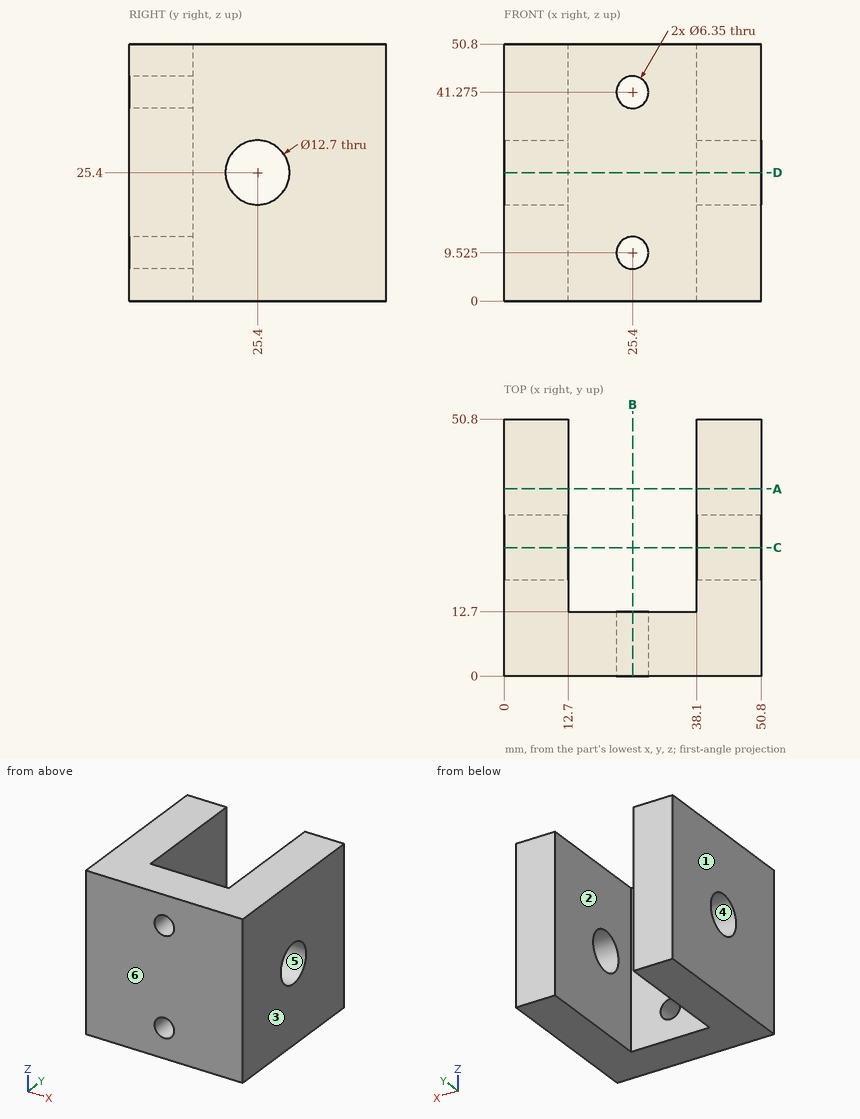
Design review of the part shown in the three views and the two pictorial views. Dimensions are in mm from the part's minimum x, y and z. A direction names the side the tool comes from. Round coordinates to 2 decimals unless told otherwise and drop trailing zeros. Write each loop counter-clockwise with the first axis right and the second up, starting at its lowest first coordinate (ties: lowest second). Pieces come first, ordered by that corner, then holes. Notation, with made-up numbers: M 66.25,65.5 L 88.25,65.5 A6 cw 88.25,69.5 Z; hole C -14.5,88.5 d6. An arc over 180 degrees is marked long. Use a Markdown table: item, result. Add a question column.
Q1. We need section D-D, the plane z = 25.4. State the section outline as (x, y) points, plus the area to 3 significant figures.
Q2. Insertion check: pin 1 (10 mm diameter, centred on y = 25.4, z = 25.4, fed in from -X). The pin has a flat end and moves straight along its axis. Give the tip position at first contact, or say it passes through.
Q3. We need section C-C, the plane y = 25.4. State the section outline as (x, z) points.
Q4. We need section A-A, the plane y = 37. State the section outline as (x, z) points, plus the area to 3 significant figures.
Q5. We need section B-B, the plane x = 25.4. State the section outline as (y, z) points.
Q6. The part is to be moulded in two halves that separate along Y. For the marked faces 3, 4, 5 and 6, say which applies: pulls with the +Y half, pulls with the -Y half, needs draft (parallel to the pull), parting line crosses it, or undercut.
Q7. Machinability: for the marked faces 1 and 2, which of the approach directions +Z, -Z, +X, -X, +Y, -Y give a long, thin tool a straight path to every point of the face, cutting with its end or side? Answer none if there is none.
Q8. To check wall thickness, follow line 1 (Z direction, x = 25.4, y = 2.5); line 2 (X direction, y = 22, z = 16); line 3 (Z direction, x = 4, y = 25.4). State the ranges of each line that lie inside material, in increasing order.
Findings below:
| question | item | result |
|---|---|---|
| 1 | outline | M 0,0 L 50.8,0 L 50.8,19.05 L 38.1,19.05 L 38.1,12.7 L 12.7,12.7 L 12.7,19.05 L 0,19.05 Z; M 0,31.75 L 12.7,31.75 L 12.7,50.8 L 0,50.8 Z; M 38.1,31.75 L 50.8,31.75 L 50.8,50.8 L 38.1,50.8 Z |
| 1 | area | 1,290 mm² |
| 2 | pin 1 | passes through |
| 3 | outline | M 0,0 L 12.7,0 L 12.7,19.05 L 0,19.05 Z; M 0,31.75 L 12.7,31.75 L 12.7,50.8 L 0,50.8 Z; M 38.1,0 L 50.8,0 L 50.8,19.05 L 38.1,19.05 Z; M 38.1,31.75 L 50.8,31.75 L 50.8,50.8 L 38.1,50.8 Z |
| 4 | outline | M 0,0 L 12.7,0 L 12.7,50.8 L 0,50.8 Z; M 38.1,0 L 50.8,0 L 50.8,50.8 L 38.1,50.8 Z |
| 4 | area | 1,290 mm² |
| 5 | outline | M 0,0 L 12.7,0 L 12.7,6.35 L 0,6.35 Z; M 0,12.7 L 12.7,12.7 L 12.7,38.1 L 0,38.1 Z; M 0,44.45 L 12.7,44.45 L 12.7,50.8 L 0,50.8 Z |
| 6 | face 3 | needs draft |
| 6 | face 4 | undercut |
| 6 | face 5 | undercut |
| 6 | face 6 | pulls with the -Y half |
| 7 | face 1 | +Z, -Z, -X, +Y, -Y |
| 7 | face 2 | +Z, -Z, +Y |
| 8 | line 1 | z = 0 to 6.35, 12.7 to 38.1, 44.45 to 50.8 |
| 8 | line 2 | x = 0 to 12.7, 38.1 to 50.8 |
| 8 | line 3 | z = 0 to 19.05, 31.75 to 50.8 |
